Part print with two shaded views. Sizes in mm from the minimum x, y, z corner. Round coordinates to 2 decimals unless told otherwise and drop trailing zeros. Loops run counter-clockwise (first coordinate to the right, second up) from the corner with the lowest first, then second, coordinate; pieces in that order, holes last.
(1) Probe probe 1 along Z at (x, y) = (385.5, 14.5); probe 2 along Y at (x, z) = (453.5, 23.5); probe 3 along Z at (x, y) = (171, 103.5). List the from-to ranges inside material, lowest first.
(2) Cut at C-C on y = 10.5. List the corners of the cut face in (x, z).
(3) Cut at B-B on z = 17.5. List the corners of the cut face in (x, y).
(4) Mould opens along Y. For the marked faces 1, 2 and 3 say: +Y half, -Y half, draft (parallel to the pull), parting line (faces both ways), or undercut.
(5) Flat gauge pin, fed straight in: pin 1 (2 mm diameter, centred on x = 143, y = 106, fed in from -Z). Where does the tip first touch, or does it go through?
(6) Cut at A-A on x = 333. List the corners of the cut face in (y, z), then the cut area to 3 significant figures.
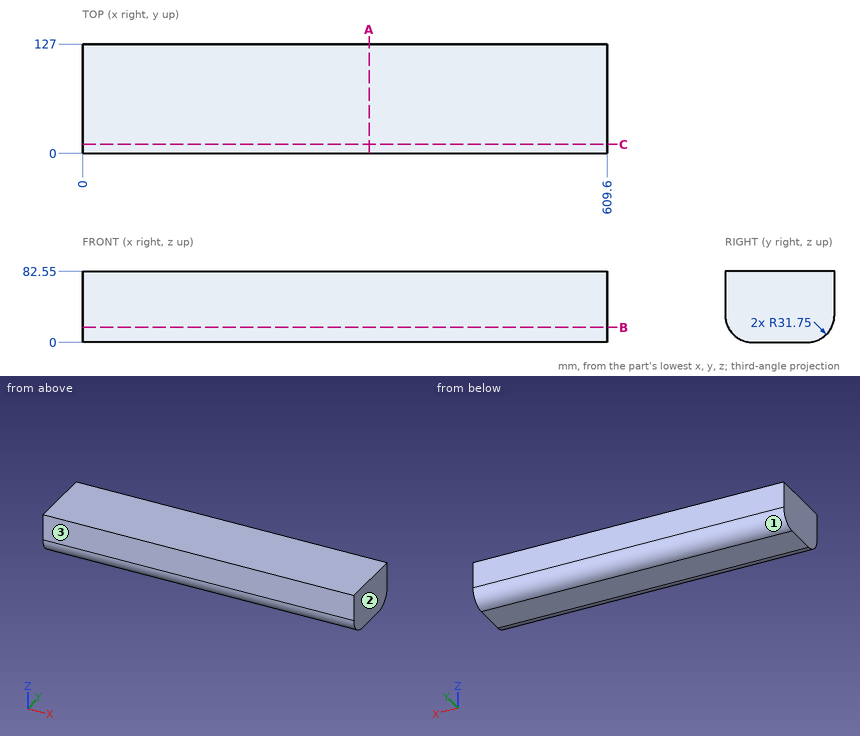
Final values:
1. probe 1: z = 5.09 to 82.55
1. probe 2: y = 1.09 to 125.91
1. probe 3: z = 1.09 to 82.55
2. outline: (0, 8.16) - (609.6, 8.16) - (609.6, 82.55) - (0, 82.55) - close
3. outline: (0, 3.38) - (609.6, 3.38) - (609.6, 123.62) - (0, 123.62) - close
4. face 1: +Y half
4. face 2: draft
4. face 3: -Y half
5. pin 1: stops at z = 1.53
6. outline: (0, 31.75) arc R31.75 ccw to (31.75, 0) - (95.25, 0) arc R31.75 ccw to (127, 31.75) - (127, 82.55) - (0, 82.55) - close
6. area: 10,100 mm2
